from build123d import *

# Parameters (mm, degrees)
ESBO_O1_W                = 126
ESBO_O1_H                = 74
ESBO_O1_W_2              = 122
ESBO_O1_H_2              = 70
RESSALTO_EXTRUS_O1_DEPTH = 60
ESBO_O2_W                = 126
ESBO_O2_H                = 74
ESBO_O2_R                = 2
RESSALTO_EXTRUS_O2_DEPTH = 2
ESBO_O3_W                = 25
ESBO_O3_H                = 25
ESBO_O3_W_2              = 14
ESBO_O3_H_2              = 16
ESBO_O3_W_3              = 10
ESBO_O3_H_3              = 30
CORTE_EXTRUS_O1_DEPTH    = 10
ESBO_O6_W                = 8
ESBO_O6_H                = 40
CORTE_EXTRUS_O2_DEPTH    = 115.214710086
ESBO_O7_W                = 10
ESBO_O7_H                = 30
CORTE_EXTRUS_O3_DEPTH    = 12
ESBO_O8_R                = 3.5
ESBO_O8_R_2              = 1.35
RESSALTO_EXTRUS_O3_DEPTH = 5


with BuildPart() as part:
    # Esboço1 → Ressalto-extrusão1 (new body)
    with BuildSketch(Plane.XY):
        Rectangle(ESBO_O1_W, ESBO_O1_H)
        Rectangle(ESBO_O1_W_2, ESBO_O1_H_2, mode=Mode.SUBTRACT)
    extrude(amount=RESSALTO_EXTRUS_O1_DEPTH)

    # Esboço2 → Ressalto-extrusão2 (add)
    with BuildSketch(Plane(origin=(0, 0, 0), x_dir=(-1, 0, 0), z_dir=(0, 0, -1))):
        Rectangle(ESBO_O2_W, ESBO_O2_H)
        with Locations((-55, -27.5)):
            Circle(ESBO_O2_R, mode=Mode.SUBTRACT)
        with Locations((55, -27.5)):
            Circle(ESBO_O2_R, mode=Mode.SUBTRACT)
        with Locations((55, 27.5)):
            Circle(ESBO_O2_R, mode=Mode.SUBTRACT)
        with Locations((-55, 27.5)):
            Circle(ESBO_O2_R, mode=Mode.SUBTRACT)
    extrude(amount=RESSALTO_EXTRUS_O2_DEPTH)

    # Esboço3 → Corte-extrusão1 (cut)
    with BuildSketch(Plane(origin=(63, 0, 0), x_dir=(0, 0, -1), z_dir=(1, 0, 0))):
        with Locations((-30.5, 19.5)):
            Rectangle(ESBO_O3_W, ESBO_O3_H)
        with Locations((-12, -15.5)):
            Rectangle(ESBO_O3_W_2, ESBO_O3_H_2)
        with Locations((-52, 0)):
            Rectangle(ESBO_O3_W_3, ESBO_O3_H_3)
    extrude(amount=-CORTE_EXTRUS_O1_DEPTH, mode=Mode.SUBTRACT)

    # Esboço6 → Corte-extrusão2 (cut, through all)
    with BuildSketch(Plane.XZ.offset(37)):
        with Locations((-49, 28)):
            Rectangle(ESBO_O6_W, ESBO_O6_H)
        with Locations((-36, 28)):
            Rectangle(ESBO_O6_W, ESBO_O6_H)
        with Locations((-23, 28)):
            Rectangle(ESBO_O6_W, ESBO_O6_H)
        with Locations((-10, 28)):
            Rectangle(ESBO_O6_W, ESBO_O6_H)
        with Locations((3, 28)):
            Rectangle(ESBO_O6_W, ESBO_O6_H)
        with Locations((16, 28)):
            Rectangle(ESBO_O6_W, ESBO_O6_H)
        with Locations((29, 28)):
            Rectangle(ESBO_O6_W, ESBO_O6_H)
        with Locations((42, 28)):
            Rectangle(ESBO_O6_W, ESBO_O6_H)
    extrude(amount=-CORTE_EXTRUS_O2_DEPTH, mode=Mode.SUBTRACT)

    # Esboço7 → Corte-extrusão3 (cut)
    with BuildSketch(Plane.ZY.offset(63)):
        with Locations((43, 0)):
            Rectangle(ESBO_O7_W, ESBO_O7_H)
        with Locations((23, 0)):
            Rectangle(ESBO_O7_W, ESBO_O7_H)
    extrude(amount=-CORTE_EXTRUS_O3_DEPTH, mode=Mode.SUBTRACT)

    # Esboço8 → Ressalto-extrusão3 (add)
    # profile 1 of 3: a face of its own
    with BuildSketch(Plane.XY):
        with Locations((-38.65, 20.4)):
            Circle(ESBO_O8_R)
        with Locations((-38.65, 20.4)):
            Circle(ESBO_O8_R_2, mode=Mode.SUBTRACT)
    # profile 2 of 3: a face of its own
    with BuildSketch(Plane.XY):
        with Locations((40.257399983, -26.445189119)):
            Circle(ESBO_O8_R)
        with Locations((40.257399983, -26.445189119)):
            Circle(ESBO_O8_R_2, mode=Mode.SUBTRACT)
    # profile 3 of 3: a face of its own
    with BuildSketch(Plane.XY):
        with Locations((41.55, 20.6)):
            Circle(ESBO_O8_R)
        with Locations((41.55, 20.6)):
            Circle(ESBO_O8_R_2, mode=Mode.SUBTRACT)
    extrude(amount=RESSALTO_EXTRUS_O3_DEPTH)


solid = part.part
Could you check a few things on this model? Use its own coordinates, in mm. A direction names the side the tool comes from. Coordinates: 2 decimals unless noted, no trailing zeros. Order: outer loops, then holes, each group sorted by start corner. A loop starts at its lowest first (then second) coordinate and runs counter-clockwise, first axis right, second up. Notation, with made-up numbers: (-28, 25.25) -> (-14, 25.25) arc R20 ccw to (-14, 43.25) -> close; hole circle Ø3 at (-13.5, -35). An arc over 180 degrees is marked (long way). One line per question, with ' | ' between items.
Q1. Thinking about a two-plate mould opening in X: for faces 1 (the face through (63, -1, 29)), 2 (the face through (-13, -37, 50)), 3 (the face through (61, -8, 30)), which applies, pulls with the +X half, pulls with the -X half, needs draft (parallel to the pull), parting line crosses it, or undercut?
Return value:
face 1: pulls with the +X half | face 2: needs draft | face 3: undercut
Q2. On a 3-axis mill with a long thin cutter (end or side, diameter ignored), from which of +Z, -Z, +X, -X, +Y, -Y can I reach the whole of each face in a straight line? I mean faces 4 (the face through (-14.4, -35, 29.6)), 5 (the face through (55.434, 25.548, -0.986)). Say none if no direction works.
Return value:
face 4: +Z | face 5: +Z, -Z
Q3. Imagine slicing it at A-A on y = 27.5. Please give me the cut outline in (x, z).
Return value:
outline: (-63, -2) -> (-57, -2) -> (-57, 0) -> (-61, 0) -> (-61, 60) -> (-63, 60) -> close; (-53, -2) -> (53, -2) -> (53, 0) -> (-53, 0) -> close; (57, -2) -> (63, -2) -> (63, 18) -> (61, 18) -> (61, 0) -> (57, 0) -> close; (61, 43) -> (63, 43) -> (63, 60) -> (61, 60) -> close
Q4. Imagine slicing it at C-C on z = 22. State how many separate pieces and enclosed holes the cut face has, and give its area (3 significant figures).
Return value:
separate pieces: 18 | enclosed holes: 0 | area: 418 mm²
Q5. If I drill on L1, parallel to Y at x = -38.65, z = 3.15; L2, parallel to Y at x = -55, z = -1; L3, parallel to X at y = -24, z = 45, over which ranges is the centre line in solid material (lowest first)?
Return value:
L1: -37 to -35, 16.9 to 19.05, 21.75 to 23.9, 35 to 37 | L2: -37 to -29.5, -25.5 to 25.5, 29.5 to 37 | L3: -63 to -61, 61 to 63
Q6. I'm going to push a flat-ended pin straight in: P1, Ø12, axis at x = 36, y = -9.5, coming from the +Z side. Where does the tip first touch, or does it pass through?
Return value:
P1: z = 0
Q7. Imagine slicing it at B-B on x = -55. Please give me the cut outline in (y, z), and give its area (3 significant figures).
Return value:
outline: (-37, -2) -> (-29.5, -2) -> (-29.5, 0) -> (-35, 0) -> (-35, 60) -> (-37, 60) -> close; (-25.5, -2) -> (25.5, -2) -> (25.5, 0) -> (-25.5, 0) -> close; (29.5, -2) -> (37, -2) -> (37, 60) -> (35, 60) -> (35, 0) -> (29.5, 0) -> close | area: 372 mm²
